```python
from build123d import *

# Parameters (mm, degrees)
F2_T = -4


with BuildPart() as f1:
    # F0 (on Front) → F1 (revolve)
    with BuildSketch(Plane.XZ):
        with BuildLine():
            Line((-16.4214689285, 60.553342104), (-13.3589282632, 0))
            Line((-13.3589282632, 0), (45.9656976163, 0))
            Line((45.9656976163, 0), (45.9656976163, 8.8407509029))
            Line((45.9656976163, 8.8407509029), (40.3396114707, 8.8407509029))
            ThreePointArc((40.3396114707, 8.8407509029), (7.5467908298, 24.8501696587), (0, 60.553342104))
            Line((0, 60.553342104), (-16.4214689285, 60.553342104))
        make_face()
    revolve(axis=Axis((-14.8901985958, 0, 30.276671052), (0.0505113539, 0, -0.9987234868)))

    # F2
    f2_openings = [f1.faces().sort_by_distance(p)[0] for p in [
        (-24.590306, 0, 59.72493),
        (-42.869881, 0, -2.992742),
    ]]
    offset(amount=F2_T, openings=f2_openings)


solid = f1.part
```
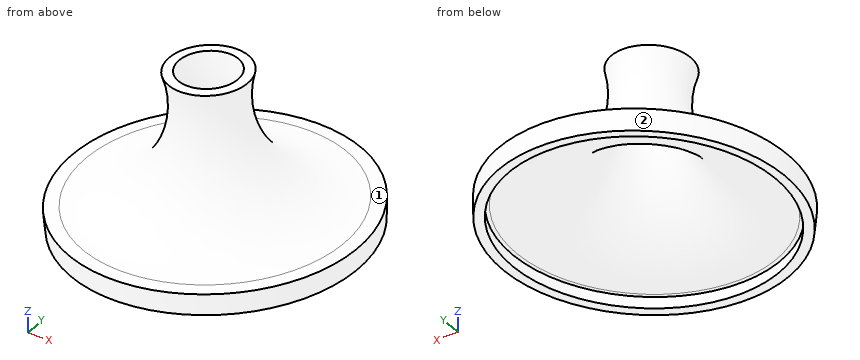
Geometry: final body of the model. Coordinates: model frame, mm. Face numbers are marked on the shaded views. A direction names the side the tool comes from. Coordinates: 2 decimals unless noted, no trailing zeros. Use CSV: the item, a comma, the result in double quotes. Start each with the question number.
1. Reachability of the marked faces 1 and 2 from +Z, -Z, +X, -X, +Y, -Y: full face, straight path, thin tool, end or side. Return the list, or none.
2. First-contact query: P1, Ø12, axis at x = 22.5, y = 18, coming from the +Z side; P2, Ø12, axis at x = -42.5, y = 6, coming from the +Z side; P3, Ø3, axis at x = 10.5, y = -6, coming from the +Z side. Flat tips, straight axial feed; report the tip coordinate or a pass-through.
3. Ray query, probe 1 along X at (y, z) = (10, 26.5) (3 decimals); probe 2 along Y at (x, z) = (-36.5, 0.5); probe 3 along X at (y, z) = (-5, 16). Return the intervals inside material, ascending.
Entries:
1,face 1,"+Z"
1,face 2,"-Z"
2,P1,"z = 13.6"
2,P2,"z = 21.91"
2,P3,"z = 22.26"
3,probe 1,"-31.87 to -26.515, -2.046 to 3.691"
3,probe 2,"-54.82 to -50.45, 50.45 to 54.82"
3,probe 3,"-41.39 to -35.95, 9.91 to 16.58"
